from build123d import *

# Parameters (mm, degrees)
SKETCH1_R           = 2.5
BOSS_EXTRUDE1_DEPTH = 4
BOSS_EXTRUDE2_START = 4
BOSS_EXTRUDE2_DEPTH = 4
SKETCH4_R           = 1.45
CUT_EXTRUDE1_DEPTH  = 4


# Read off the part's stored shape, not the designer's step: Boss-Extrude2
with BuildPart() as part:
    # Sketch1 → Boss-Extrude1 (new body)
    with BuildSketch(Plane(origin=(0, 0, 0), x_dir=(1, 0, 0), z_dir=(0, 1, 0))):
        Polygon((-4.5, -4.5), (45.5, -4.5), (90.417468245, 21.433112383), (97.448557159, 17.373711306), (110.438938215, 24.873711306), (106.438938215, 27.183112383), (104.376760389, 25.992513459), (97.448557159, 21.992513459), (90.520353928, 25.992513459), (90.520353928, 33.992513459), (99.510734985, 39.183112383), (99.510734985, 43.801914536), (86.520353928, 36.301914536), (86.520353928, 28.183112383), (45.5, 4.5), (-4.5, 4.5), align=None)
        with Locations(Location((0, 0, 0), (0, 0, 270))):
            Circle(SKETCH1_R, mode=Mode.SUBTRACT)
    extrude(amount=BOSS_EXTRUDE1_DEPTH)

    # Boss-Extrude2 outline → Boss-Extrude2 (add)
    with BuildSketch(Plane(origin=(0, 0, 0), x_dir=(1, 0, 0), z_dir=(0, 1, 0)).offset(BOSS_EXTRUDE2_START)):
        Polygon((99.510734985, 39.183112383), (99.510734985, 43.801914536), (86.520353928, 36.301914536), (86.520353928, 28.183112383), (45.5, 4.5), (-4.5, 4.5), (-4.5, -4.5), (45.5, -4.5), (90.417468245, 21.433112383), (97.448557159, 17.373711306), (110.438938215, 24.873711306), (106.438938215, 27.183112383), (97.448557159, 21.992513459), (90.520353928, 25.992513459), (90.520353928, 33.992513459), align=None)
    extrude(amount=BOSS_EXTRUDE2_DEPTH)

    # Sketch4 → Cut-Extrude1 (cut)
    with BuildSketch(Plane(origin=(5.910898385, 0, 10.237976321), x_dir=(-0.8660254037844413, 0, 0.4999999999999956), z_dir=(-0.4999999999999956, 0, -0.8660254037844413))):
        with Locations((-103.079781714, 4)):
            Circle(SKETCH4_R)
    extrude(amount=-CUT_EXTRUDE1_DEPTH, mode=Mode.SUBTRACT)


solid = part.part
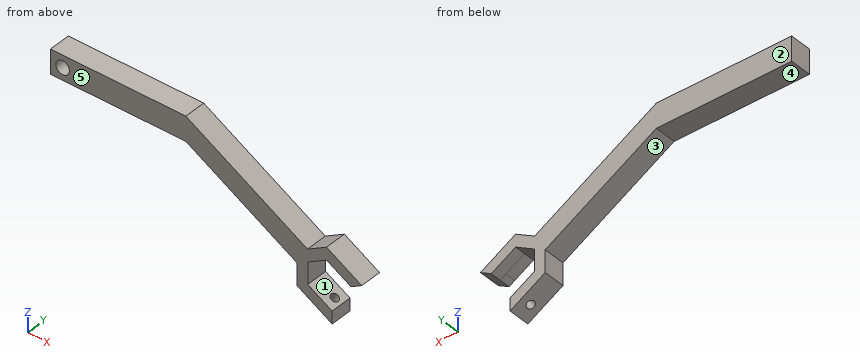
Input: part model. Units: mm. Frame: model coordinates. Face numbers are marked on the shaded views. A direction names the side the tool comes from. Coordinates: 2 decimals unless noted, no trailing zeros. Loops run counter-clockwise (first coordinate to the right, second up) from the corner with the lowest first, then second, coordinate; pieces in that order, holes last.
(1) Set-up query: the marked faces 4 and 5. Return all of +Z, -Z, +X, -X, +Y, -Y with unobstructed straight access to the full face (end or side cutting, diameter ignored); none if empty.
(2) Section D-D on x = 51.5. Return the cut outline in (y, z).
(3) Section B-B on z = 0. Return the cut outline in (x, y), then the cut area to 3 significant figures.
(4) First-contact query: pin 1 Ø2 at (x, y) = (51, 4.5) entering from -Z; pin 2 Ø3 at (y, z) = (5, -34) entering from +X; pin 3 Ø3.5 at (y, z) = (3.5, -40.5) entering from +X. Flat tips, straight axial feed; report the tip coordinate or a pass-through.
(5) Pull-direction query (Z, two-part tool) for the marked faces 1, 2 and 3; classes: released by +Z, released by -Z, zero draft, split by the parting line, or undercut.
(6) Section A-A on x = 0. Return the cut outline in (y, z), then the cut area to 3 significant figures.
(7) Section C-C on z = -31. Return the cut outline in (x, y).
(8) Material intervals for probe 1 along X at (y, z) = (1.15, 0); probe 2 along X at (y, z) = (3.5, 1.5); probe 3 along X at (y, z) = (3.5, -33.5), sorted ascending.
Data:
1. face 4: -Z, -X, +Y, -Y
1. face 5: +Z, -Z, +X, -X, -Y
2. outline: (0, -7.96) - (8, -7.96) - (8, 1.04) - (0, 1.04) - close
3. outline: (-4.5, 0) - (-2.5, 0) - (-2.5, 4) - (2.5, 4) - (2.5, 0) - (53.29, 0) - (53.29, 8) - (-4.5, 8) - close
3. area: 442 mm2
4. pin 1: stops at z = -8.25
4. pin 2: stops at x = 93.13
4. pin 3: stops at x = 99.51
5. face 1: undercut
5. face 2: zero draft
5. face 3: released by -Z
6. outline: (0, -4.5) - (8, -4.5) - (8, 4.5) - (0, 4.5) - (0, 2.5) - (4, 2.5) - (4, -2.5) - (0, -2.5) - close
6. area: 52.0 mm2
7. outline: (86.52, 0) - (90.52, 0) - (90.52, 8) - (86.52, 8) - close
8. probe 1: x = -4.5 to -2.5, 2.5 to 53.29
8. probe 2: x = -4.5 to -2, 2 to 50.7
8. probe 3: x = 86.52 to 90.52
